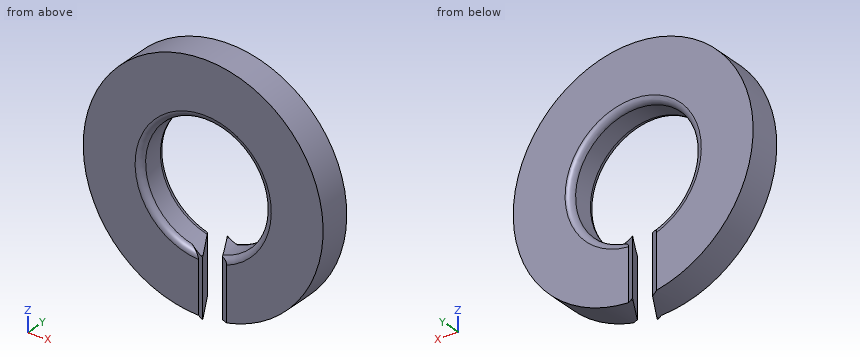
```python
from build123d import *

# Parameters (mm, degrees)
BODYSKE_W       = 2.85
BODYSKE_H       = 20
CUT_EXTRASKE_W  = 11.8
CUT_EXTRASKE_H  = 9.2
CUT_EXTRA_DEPTH = 14.023824323
TYPE_A_DEPTH    = 14.023824323
FILLET1_R       = 0.3


with BuildPart() as part:
    # BodySke → BaseBody (revolve)
    with BuildSketch(Plane.XY, mode=Mode.PRIVATE) as basebody_sk:
        with Locations((4.475, 0)):
            Rectangle(BODYSKE_W, BODYSKE_H)
    revolve(basebody_sk.sketch.rotate(Axis((0, 0, 0), (0, 1, 0)), 90), axis=Axis((0, 0, 0), (0, 1, 0)))

    # Cut-ExtraSke → Cut-Extra (cut, through all)
    with BuildSketch(Plane.XY):
        with Locations((0, -5.4)):
            Rectangle(CUT_EXTRASKE_W, CUT_EXTRASKE_H)
        with Locations((0, 5.4)):
            Rectangle(CUT_EXTRASKE_W, CUT_EXTRASKE_H)
    extrude(amount=CUT_EXTRA_DEPTH, mode=Mode.SUBTRACT)

    # ASke → Type-A (cut, through all)
    with BuildSketch(Plane.XY):
        Polygon((0.115470054, -1), (-0.230940108, -0.8), (-5.9, -0.8), (-5.9, -10), (5.9, -10), (5.9, -0.8), (1.154700538, -0.8), (0.808290377, -0.6), (-0.115470054, 1), (0.230940108, 0.8), (5.9, 0.8), (5.9, 10), (-5.9, 10), (-5.9, 0.8), (-1.154700538, 0.8), (-0.808290377, 0.6), align=None)
    extrude(amount=-TYPE_A_DEPTH, mode=Mode.SUBTRACT)

    # Fillet1
    fillet1_edges = [part.edges().sort_by_distance(p)[0] for p in [
        (-0.474598894, -0.8, 3.012848468),
        (0.474598894, 0.8, 3.012848468),
    ]]
    fillet(fillet1_edges, radius=FILLET1_R)


solid = part.part
```
For this review, take the finished solid that the model builds, in its own axes (mm). Round coordinates to 2 decimals unless told otherwise and drop trailing zeros. Order: outer loops, then holes, each group sorted by start corner. A loop starts at its lowest first (then second) coordinate and runs counter-clockwise, first axis right, second up.
Q1. Wall thickness on line 1 (X direction, y = -0.55, z = 0); line 2 (Z direction, x = -2.5, y = 0.15): over which ranges is each line inside the solid? List them lowest first.
Findings below:
line 1: x = -5.9 to -3.05, 3.05 to 5.9
line 2: z = -5.34 to -1.75, 1.75 to 5.34
Q2. We need section A-A, the plane z = -4. Give the boundary of the cut face in (x, y).
Findings below:
outline: (-4.34, -0.8) - (-0.23, -0.8) - (0.12, -1) - (-0.81, 0.6) - (-1.15, 0.8) - (-4.34, 0.8) - close; (-0.12, 1) - (0.81, -0.6) - (1.15, -0.8) - (4.34, -0.8) - (4.34, 0.8) - (0.23, 0.8) - close
Q3. We need section B-B, the plane z = 0. Give the boundary of the cut face in (x, y).
Findings below:
outline: (-5.9, -0.8) - (-3.35, -0.8) arc R0.3 ccw to (-3.05, -0.5) - (-3.05, 0.5) arc R0.3 ccw to (-3.35, 0.8) - (-5.9, 0.8) - close; (3.05, -0.5) arc R0.3 ccw to (3.35, -0.8) - (5.9, -0.8) - (5.9, 0.8) - (3.35, 0.8) arc R0.3 ccw to (3.05, 0.5) - close
Q4. Insertion check: P1, Ø1, axis at x = 1, z = 1.5, coming from the +Y side; P2, Ø5, axis at x = -2, z = -1, coming from the +Y side; P3, Ø3.5, axis at x = -2, z = 1, coming from the -Y side. Each pin has a flat end and moves straight along its axis. Give the tip position at first contact, or say it passes through.
Findings below:
P1: passes through
P2: stops at y = 0.8
P3: stops at y = -0.8
Q5. We need section D-D, the plane z = 4. Give the boundary of the cut face in (x, y), plus the area to 3 significant figures.
Findings below:
outline: (-4.34, -0.8) - (4.34, -0.8) - (4.34, 0.8) - (-4.34, 0.8) - close
area: 13.9 mm2
Q6. We need section C-C, the plane x = -4.5. Give the boundary of the cut face in (y, z), plus the area to 3 significant figures.
Findings below:
outline: (-0.8, -3.82) - (0.8, -3.82) - (0.8, 3.82) - (-0.8, 3.82) - close
area: 12.2 mm2
